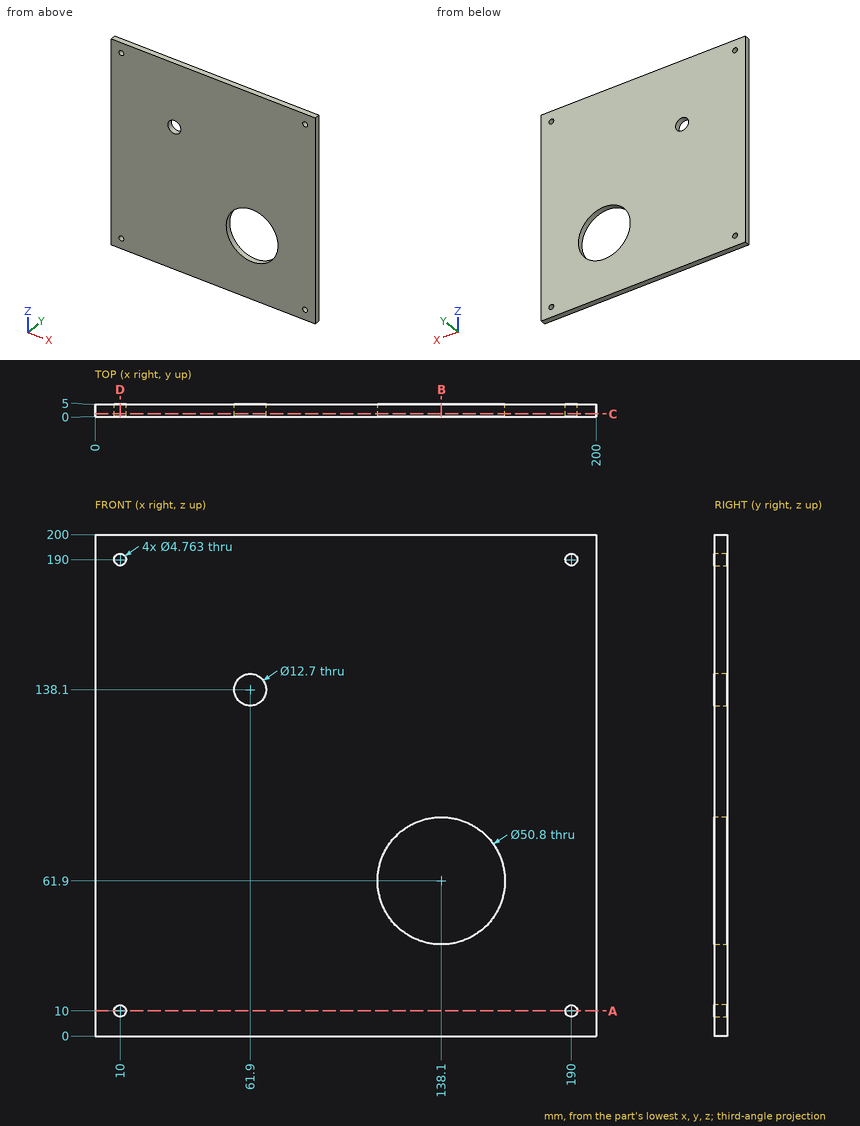
Design review of the part shown in the three views and the two pictorial views. Dimensions are in mm from the part's minimum x, y and z. Give positions to 0.01 mm unless a question says otherwise; leave off trailing zeros. Order: outer loops, then holes, each group sorted by start corner. A loop starts at its lowest first (then second) coordinate and runs counter-clockwise, first axis right, second up. Notation, with made-up numbers: M -0.75,-10 L 17.25,-10 A19 cw 17.25,21 Z; hole C 45.25,82.5 d6. An arc over 180 degrees is marked long. Answer in a Markdown table with one row per item. Add a question column.
(1) Consider section A-A on z = 10. State the section outline as (x, y) points.
(2) Consider section C-C on y = 1.05. State the section outline as (x, z) points, and give its area (3 significant figures).
(3) Consider section B-B on x = 138.1. State the section outline as (y, z) points, and give its area (3 significant figures).
(4) Consider section D-D on x = 10. State the section outline as (y, z) points.
(5) Wall thickness on probe 1 along X at (y, z) = (1.55, 190); probe 2 along Z at (x, y) = (138, 1.1); probe 3 along X at (y, z) = (2.85, 61.9): over which ranges is each line inside the solid? List them lowest first. Write a range as [from, to].
Evaluation:
| question | item | result |
|---|---|---|
| 1 | outline | M 0,0 L 7.62,0 L 7.62,5 L 0,5 Z; M 12.38,0 L 187.62,0 L 187.62,5 L 12.38,5 Z; M 192.38,0 L 200,0 L 200,5 L 192.38,5 Z |
| 2 | outline | M 0,0 L 200,0 L 200,200 L 0,200 Z; hole C 10,10 d4.76; hole C 10,190 d4.76; hole C 61.9,138.1 d12.7; hole C 138.1,61.9 d50.8; hole C 190,10 d4.76; hole C 190,190 d4.76 |
| 2 | area | 37,800 mm^2 |
| 3 | outline | M 0,0 L 5,0 L 5,36.5 L 0,36.5 Z; M 0,87.3 L 5,87.3 L 5,200 L 0,200 Z |
| 3 | area | 746 mm^2 |
| 4 | outline | M 0,0 L 5,0 L 5,7.62 L 0,7.62 Z; M 0,12.38 L 5,12.38 L 5,187.62 L 0,187.62 Z; M 0,192.38 L 5,192.38 L 5,200 L 0,200 Z |
| 5 | probe 1 | x = [0, 7.62], [12.38, 187.62], [192.38, 200] |
| 5 | probe 2 | z = [0, 36.5], [87.3, 200] |
| 5 | probe 3 | x = [0, 112.7], [163.5, 200] |
